Solid Edge part; units mm, degrees
sketch "Sketch1" plane through (0, 0, 0) normal (0, -1, 0) x (1, 0, 0)
  circle A0 centre (0, 0) radius 39.5
extrude "Protrusion1" add sketch "Sketch1" against normal blind 14
sketch "Sketch2" plane through (0, 0, 0) normal (0, -1, 0) x (1, 0, 0)
  circle A0 centre (0, 0) radius 25
extrude "Cutout1" cut sketch "Sketch2" against normal up to next
sketch "Sketch3" plane through (0, 0, 0) normal (1, 0, 0) x (0, 1, 0)
  line L0 (2, 39.5) -> (4.7516, 30.5)
  line L1 (4.7516, 30.5) -> (9.2484, 30.5)
  line L2 (9.2484, 30.5) -> (12, 39.5)
  line L3 (12, 39.5) -> (2, 39.5)
revolve "RevolvedCutout1" cut sketch "Sketch3" angle 360 about axis through (0, 0, 0) along (0, 1, 0)
properties material "Steel"
Model file for the job. Use its own axes, mm. A direction names the side the tool comes from. Give positions to 0.01 mm unless a question says otherwise; leave off trailing zeros. Loops run counter-clockwise (first coordinate to the right, second up) from the corner with the lowest first, then second, coordinate; pieces in that order, holes last.
Item 1: Slice it at B-B (z = 0). Write the cut outline in (x, y).
Check values:
outline: (-39.5, 0) - (-25, 0) - (-25, 14) - (-39.5, 14) - (-39.5, 12) - (-30.5, 9.25) - (-30.5, 4.75) - (-39.5, 2) - close; (25, 0) - (39.5, 0) - (39.5, 2) - (30.5, 4.75) - (30.5, 9.25) - (39.5, 12) - (39.5, 14) - (25, 14) - close
Item 2: Which spindle directions (+Z, -Z, +X, -X, +Y, -Y) get a long thin tool onto all of the face, cutting with end or side? Do faces 4 (the face through (-26, 14, 1)), 5 (the face through (-9.33, 4.58, 29.63)). Say none if no direction does.
Check values:
face 4: +Z, -Z, +X, -X, +Y
face 5: none
Item 3: Slice it at C-C (y = 10.5). Write the cut outline in (x, z).
Check values:
outline: circle Ø69.19 at (0, 0); hole circle Ø50 at (0, 0)
Item 4: Drop flat-ended pins along their axis: P1, Ø8, axis at y = 2, z = -30.5, coming from the +X side; P2, Ø3, axis at x = 22.5, y = 2.5, coming from the -Z side; P3, Ø2, axis at x = 8.5, y = 12, coming from the +Z side. Give the stop position or say it passes through.
Check values:
P1: stops at x = 29.29
P2: stops at z = -33.4
P3: stops at z = 38.78
Item 5: Slice it at A-A (x = 0). Write the cut outline in (y, z), plus the area to 3 significant figures.
Check values:
outline: (0, -39.5) - (2, -39.5) - (4.75, -30.5) - (9.25, -30.5) - (12, -39.5) - (14, -39.5) - (14, -25) - (0, -25) - close; (0, 25) - (14, 25) - (14, 39.5) - (12, 39.5) - (9.25, 30.5) - (4.75, 30.5) - (2, 39.5) - (0, 39.5) - close
area: 276 mm2
Item 6: Mould opens along Y. For faces 1 (the face through (23.846, 6.902, 7.509)), 2 (the face through (-30.32, 9.42, -6.73)), 3 (the face through (-26, 0, 1)) say: +Y half, -Y half, draft (parallel to the pull), parting line (faces both ways), or undercut.
Check values:
face 1: draft
face 2: undercut
face 3: -Y half
Item 7: Drill centre lines: line 1 along Y through (x, z) = (4.5, -34); line 2 along Y through (x, z) = (30, 24); line 3 along Z through (x, y) = (-21, 6.5). Where is each one in solid material? Low to high.
Check values:
line 1: y = 0 to 3.59, 10.41 to 14
line 2: y = 0 to 2.33, 11.67 to 14
line 3: z = -22.12 to -13.56, 13.56 to 22.12
Item 8: Slice it at D-D (y = 3.75). Write the cut outline in (x, z).
Check values:
outline: circle Ø67.55 at (0, 0); hole circle Ø50 at (0, 0)
